Autodesk Inventor part; units mm, degrees
ref_plane "YZ Plane" through (0, 0, 0) normal (1, 0, 0) x (0, 1, 0)
ref_plane "XZ Plane" through (0, 0, 0) normal (0, 1, 0) x (-1, 0, 0)
ref_plane "XY Plane" through (0, 0, 0) normal (0, 0, 1) x (1, 0, 0)
sketch "スケッチ1" plane through (0, 0, 0) normal (1, 0, 0) x (0, 1, 0)
  line L0 (0, 0) -> (31.7, 0)
  line L1 (1.7, 14) -> (30, 14)
  line L2 (1.7, 14) -> (0, 0)
  line L3 (30, 14) -> (31.7, 0)
  dimension "d0" = 31.7
  dimension "d1" = 28.3
extrude "押し出し1" add sketch "スケッチ1" against normal blind 24
sketch "スケッチ2" plane through (-24, 0, 0) normal (-1, 0, 0) x (0, 0, 1)
  line L0 (0, 0) -> (14, 1.7)
  line L1 (3, 0.3643) -> (3, 31.3357)
  line L2 (14, 30) -> (0, 31.7)
  line L3 (4.3, 0.3643) -> (4.3, 31.3357)
  line L4 (4.3, 31.3357) -> (3, 31.3357)
  line L5 (4.3, 0.3643) -> (3, 0.3643)
  point P0 (4.3, 0.5221)
  point P1 (4.3, 31.1779)
extrude "押し出し2" cut sketch "スケッチ2" against normal blind 21 contours L1 L2 L3 L0
sketch "スケッチ4" plane through (-3, 0, 0) normal (-1, 0, 0) x (0, 0, 1)
  circle A0 centre (9, 9.85) radius 1.75
  circle A1 centre (9, 21.85) radius 1.75
  point P0 (0, 0)
  dimension "d10" = 3.5
  dimension "d11" = 3.5
extrude "押し出し4" cut sketch "スケッチ4" along normal mid plane 100
fillet "フィレット1" radius 3 2 edges at (0, 30.85, 7) (0, 0.85, 7)
sketch "スケッチ10" plane through (-24, 0, 0) normal (-1, 0, 0) x (0, 0, 1)
  line L0 (5.6, 13.45) -> (12.4, 13.45)
  line L1 (12.4, 13.45) -> (12.4, 18.25)
  line L2 (12.4, 18.25) -> (5.6, 18.25)
  line L3 (5.6, 18.25) -> (5.6, 13.45)
  line L4 (5.6, 13.45) -> (12.4, 18.25) construction
  line L5 (12.4, 13.45) -> (5.6, 18.25) construction
  line L6 (14, 1.7) -> (14, 30)
  point P0 (0, 0)
  point P1 (9, 15.85)
  point P2 (14, 15.85)
  dimension "d29" = 6.8
  dimension "d30" = 4.8
  dimension "d44" = 5
extrude "押し出し10" add sketch "スケッチ10" along normal blind 3
sketch "スケッチ11" plane through (-24, 0, 0) normal (-1, 0, 0) x (0, 0, 1)
  line L0 (12.3, 3.2) -> (5.5, 3.2)
  line L1 (5.5, 3.2) -> (5.5, 6)
  line L2 (5.5, 6) -> (12.3, 6)
  line L3 (12.3, 6) -> (12.3, 3.2)
  line L4 (12.3, 3.2) -> (5.5, 6) construction
  line L5 (5.5, 3.2) -> (12.3, 6) construction
  line L6 (12.3, 28.5) -> (5.5, 28.5)
  line L7 (5.5, 28.5) -> (5.5, 25.7)
  line L8 (5.5, 25.7) -> (12.3, 25.7)
  line L9 (12.3, 25.7) -> (12.3, 28.5)
  line L10 (12.3, 28.5) -> (5.5, 25.7) construction
  line L11 (5.5, 28.5) -> (12.3, 25.7) construction
  point P0 (0, 0)
  point P1 (8.9, 4.6)
  point P2 (8.9, 27.1)
  dimension "d33" = 6.8
  dimension "d34" = 2.8
  dimension "d35" = 6.8
  dimension "d36" = 2.8
extrude "押し出し11" add sketch "スケッチ11" along normal blind 3
sketch "スケッチ12" plane through (-24, 0, 0) normal (-1, 0, 0) x (0, 0, 1)
  line L0 (2.05, 24.15) -> (0.75, 24.15)
  line L1 (0.75, 24.15) -> (0.75, 19.35)
  line L2 (0.75, 19.35) -> (2.05, 19.35)
  line L3 (2.05, 19.35) -> (2.05, 24.15)
  line L4 (2.05, 24.15) -> (0.75, 19.35) construction
  line L5 (0.75, 24.15) -> (2.05, 19.35) construction
  line L6 (0.75, 7.45) -> (2.05, 7.45)
  line L7 (2.05, 7.45) -> (2.05, 12.25)
  line L8 (2.05, 12.25) -> (0.75, 12.25)
  line L9 (0.75, 12.25) -> (0.75, 7.45)
  line L10 (0.75, 7.45) -> (2.05, 12.25) construction
  line L11 (2.05, 7.45) -> (0.75, 12.25) construction
  point P0 (0, 0)
  point P1 (1.4, 21.75)
  point P2 (1.4, 9.85)
  dimension "d39" = 1.3
  dimension "d40" = 4.8
  dimension "d45" = 1.3
  dimension "d46" = 4.8
extrude "押し出し12" add sketch "スケッチ12" along normal blind 3 contours L3 L2 L1 L0
sketch "スケッチ13" plane through (-24, 0, 0) normal (-1, 0, 0) x (0, 0, 1)
  line L0 (2.05, 12.25) -> (0.75, 12.25)
  line L1 (0.75, 12.25) -> (0.75, 7.45)
  line L2 (0.75, 7.45) -> (2.05, 7.45)
  line L3 (2.05, 7.45) -> (2.05, 12.25)
  line L4 (2.05, 12.25) -> (0.75, 7.45) construction
  line L5 (0.75, 12.25) -> (2.05, 7.45) construction
  point P0 (0, 0)
  point P1 (1.4, 9.85)
  dimension "d47" = 1.3
  dimension "d48" = 4.8
extrude "押し出し13" add sketch "スケッチ13" along normal blind 3
properties part number "finlay_holds_down" material "ABS プラスチック"
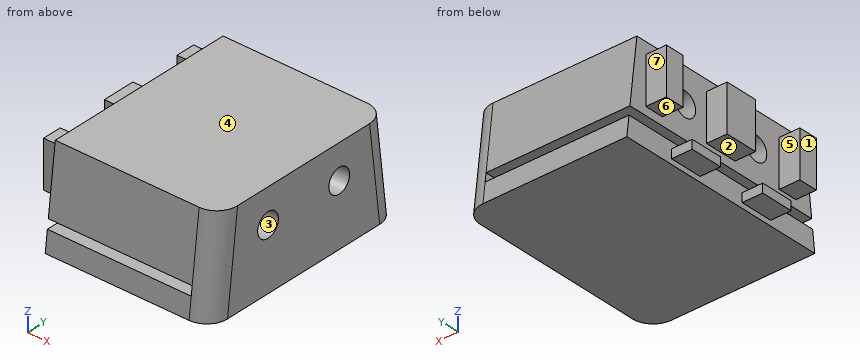
CAD build for the part. Positions are in the model's coordinates, mm. Face numbers are marked on the shaded views. A direction names the side the tool comes from. Round coordinates to 2 decimals unless told otherwise and drop trailing zeros. Order: outer loops, then holes, each group sorted by start corner. A loop starts at its lowest first (then second) coordinate and runs counter-clockwise, first axis right, second up. Notation, with made-up numbers: (75.5, 76) - (129.5, 76) arc R24 ccw to (129.5, 108) - close; hole circle Ø8 at (32, -23.75). An arc over 180 degrees is marked (long way). Use CSV: the item, a comma, the result in double quotes. Start each with the question number.
1) Two-plate mould, pull along Z, no slides. Class the marked faces 1, 2 and 3: pulls with the +Z half, pulls with the -Z half, needs draft (parallel to the pull), parting line crosses it, or undercut.
2) Saw through at A-A (x = -21). List the corners of the cut face in (y, z), and give its area (3 significant figures).
3) Tool access for the marked faces 4, 5, 6 and 7: list every direction of +Z, -Z, +X, -X, +Y, -Y with a clear straight run to the whole face (end or side of a thin tool).
4) Pin check, flat tips, straight feed: pin 1 Ø3.5 at (x, y) = (-26, 22.5) entering from +Z; pin 2 Ø5 at (x, y) = (-19, 26.5) entering from -Z; pin 3 Ø0.9 at (x, y) = (-26, 22) entering from -Z; pin 4 Ø0.9 at (x, z) = (-25.5, 10.5) entering from +Y. Stop position of each tip, or through.
5) Saw through at B-B (y = 9.85). List the corners of the cut face in (x, z).
6) Saw through at C-C (y = 25). List the corners of the cut face in (x, z).
7) Saw through at D-D (z = 9). Count the separate pieces of the cut face and the enclosed holes in it, and give its area (3 significant figures).
8) Wall check: L1, parallel to Z at x = -9, y = 9.85; L2, parallel to Z at x = -9, y = 14.5; L3, parallel to Y at x = -5.5, z = 9. Give the ranges that are in metal, low to high. Write a range as [from, to].
Values follow:
1,face 1,"needs draft"
1,face 2,"pulls with the -Z half"
1,face 3,"undercut"
2,outline,"(0, 0) - (31.7, 0) - (31.34, 3) - (0.36, 3) - close; (0.52, 4.3) - (31.18, 4.3) - (30, 14) - (1.7, 14) - close; hole circle Ø3.5 at (9.85, 9); hole circle Ø3.5 at (21.85, 9)"
2,area,"361 mm2"
3,face 4,"+Z, +X, -X, +Y, -Y"
3,face 5,"+Z, -Z, -X"
3,face 6,"-Z, -X, +Y, -Y"
3,face 7,"+Z, -Z, -X, +Y"
4,pin 1,"stops at z = 2.05"
4,pin 2,"stops at z = 0"
4,pin 3,"stops at z = 0.75"
4,pin 4,"stops at y = 28.5"
5,outline,"(-27, 0.75) - (-24, 0.75) - (-24, 0) - (0, 0) - (0, 7.25) - (-24, 7.25) - (-24, 4.3) - (-3, 4.3) - (-3, 3) - (-24, 3) - (-24, 2.05) - (-27, 2.05) - close; (-24, 10.75) - (0, 10.75) - (0, 14) - (-24, 14) - close"
6,outline,"(-24, 0) - (0, 0) - (0, 14) - (-24, 14) - (-24, 4.3) - (-3, 4.3) - (-3, 3) - (-24, 3) - close"
7,separate pieces,"3"
7,enclosed holes,"0"
7,area,"568 mm2"
8,L1,"z = [0, 3], [4.3, 7.25], [10.75, 14]"
8,L2,"z = [0, 3], [4.3, 14]"
8,L3,"y = [1.09, 8.1], [11.6, 20.1], [23.6, 30.61]"
